Check sheet for the modelled part. Datum: model origin and axes. Units: mm. A direction names the side the tool comes from. Coordinates: 2 decimals unless noted, no trailing zeros. Order: outer loops, then holes, each group sorted by start corner. A loop starts at its lowest first (then second) coordinate and runs counter-clockwise, first axis right, second up.
1. Set-up check for faces 5 (the flat face through (15, 1, 1)), 6 (the flat face through (54, 45, 1)), 7 (the flat face through (32.5, 99, 1)): record each of +Z, -Z, +X, -X, +Y, -Y from which the full face is reachable in a straight line by a thin tool's end or side.
2. Cross-section at C-C (y = 33.75). Enter the section's corners in (x, z).
3. Cross-section at A-A (y = 78). Enter the section's corners in (x, z).
4. Cross-section at D-D (z = 0.55). Count the separate pieces of the cut face and the enclosed holes in it, then the cut area to 3 significant figures.
5. Gauge pin test, flat ends, axial feed: pin 1 Ø0.6 at (x, z) = (34, 1) entering from +Y; pin 2 Ø2 at (x, y) = (47.25, 33.75) entering from -Z; pin 3 Ø0.6 at (x, z) = (1, 1) entering from -Y; pin 4 Ø1 at (x, z) = (32, 1.5) entering from -Y. Record the tip position at first contact, or that the pin passes through.
6. Thickness scan on line 1 (Y direction, x = 23.75, z = 0.95); line 2 (X direction, y = 92.25, z = 1.6); line 3 (X direction, y = 47, z = 0.25). Record the ranges inside material, lowest first.
7. Cross-section at B-B (x = 12). Enter the section's corners in (y, z), then the cut area to 3 significant figures.
8. Draft check along X on faces 1 (the flat face through (27, 2, 1)), 2 (the flat face through (1, 45, 1)), 3 (the flat face through (53, 22, 1)), 4 (the flat face through (22.5, 99, 1)). Enter one of: released by +X, released by -X, zero draft, split by the parting line, or undercut.
```python
from build123d import *

# Parameters (mm, degrees)
SKETCH1_R           = 1.25
SKETCH1_R_2         = 3.5
SKETCH1_W           = 2
SKETCH1_H           = 10
BOSS_EXTRUDE1_DEPTH = 2


with BuildPart() as part:
    # Sketch1 → Boss-Extrude1 (new body)
    with BuildSketch(Plane.XY):
        Polygon((22.5, 100), (22.5, 98), (2, 98), (2, 55), (0, 55), (0, 45), (2, 45), (2, 0), (15, 0), (15, 2), (40, 2), (40, 0), (53, 0), (53, 45), (55, 45), (55, 55), (53, 55), (53, 98), (32.5, 98), (32.5, 100), align=None)
        with Locations((47.25, 92.25)):
            Circle(SKETCH1_R, mode=Mode.SUBTRACT)
        with Locations((23.75, 92.25)):
            Circle(SKETCH1_R, mode=Mode.SUBTRACT)
        with Locations((47.25, 33.75)):
            Circle(SKETCH1_R, mode=Mode.SUBTRACT)
        with Locations((23.75, 33.75)):
            Circle(SKETCH1_R, mode=Mode.SUBTRACT)
        with Locations((12, 78)):
            Circle(SKETCH1_R_2, mode=Mode.SUBTRACT)
        with Locations((34, 50)):
            Rectangle(SKETCH1_W, SKETCH1_H, mode=Mode.SUBTRACT)
    extrude(amount=BOSS_EXTRUDE1_DEPTH)


solid = part.part
```
Data:
1. face 5: +Z, -Z, -Y
1. face 6: +Z, -Z, +X, -Y
1. face 7: +Z, -Z, +X, +Y
2. outline: (2, 0) - (22.5, 0) - (22.5, 2) - (2, 2) - close; (25, 0) - (46, 0) - (46, 2) - (25, 2) - close; (48.5, 0) - (53, 0) - (53, 2) - (48.5, 2) - close
3. outline: (2, 0) - (8.5, 0) - (8.5, 2) - (2, 2) - close; (15.5, 0) - (53, 0) - (53, 2) - (15.5, 2) - close
4. separate pieces: 1
4. enclosed holes: 6
4. area: 4,930 mm2
5. pin 1: stops at y = 98
5. pin 2: passes through
5. pin 3: stops at y = 45
5. pin 4: stops at y = 2
6. line 1: y = 2 to 32.5, 35 to 91, 93.5 to 100
6. line 2: x = 2 to 22.5, 25 to 46, 48.5 to 53
6. line 3: x = 0 to 33, 35 to 55
7. outline: (0, 0) - (74.5, 0) - (74.5, 2) - (0, 2) - close; (81.5, 0) - (98, 0) - (98, 2) - (81.5, 2) - close
7. area: 182 mm2
8. face 1: undercut
8. face 2: zero draft
8. face 3: released by +X
8. face 4: released by -X
